from build123d import *

# Parameters (mm, degrees)
EXTRUDE_1_DEPTH     = 38
SKETCH_2_R          = 5
SKETCH_2_W          = 10
SKETCH_2_H          = 19
CUT_EXTRUDE_1_DEPTH = 8
SKETCH_3_W          = 4
SKETCH_3_H          = 4
CUT_EXTRUDE_2_DEPTH = 51.970579749
CUT_EXTRUDE_3_DEPTH = 65.567793829


with BuildPart() as part:
    # Эскиз1 → Бобышка-Вытянуть1 (new body)
    with BuildSketch(Plane.XY):
        Polygon((-5, 0), (-25, 0), (-25, -15), (25, -15), (25, 15), (12, -8), (-5, -8), align=None)
    extrude(amount=EXTRUDE_1_DEPTH)

    # Эскиз2 → Вырез-Вытянуть1 (cut)
    with BuildSketch(Plane(origin=(0, 0, 0), x_dir=(1, 0, 0), z_dir=(0, 1, 0))):
        with Locations((-25, -9.5)):
            Circle(SKETCH_2_R)
        with Locations((-10, -28.5)):
            Rectangle(SKETCH_2_W, SKETCH_2_H)
    extrude(amount=-CUT_EXTRUDE_1_DEPTH, mode=Mode.SUBTRACT)

    # Эскиз3 → Вырез-Вытянуть2 (cut, through all)
    with BuildSketch(Plane(origin=(0, -8, 0), x_dir=(1, 0, 0), z_dir=(0, 1, 0))):
        with Locations((-25, -9.5)):
            Rectangle(SKETCH_3_W, SKETCH_3_H)
        Polygon((1.350852961, -27), (7.701705922, -38), (-5, -38), align=None)
    extrude(amount=-CUT_EXTRUDE_2_DEPTH, mode=Mode.SUBTRACT)

    # Эскиз4 → Вырез-Вытянуть3 (cut, through all)
    with BuildSketch(Plane(origin=(25, 0, 0), x_dir=(0, 0, -1), z_dir=(1, 0, 0))):
        Polygon((-8, 15), (-28, 15), (-28, 5), (-8, 5), (-8, 10), (0, 10), (0, 15), align=None)
    extrude(amount=-CUT_EXTRUDE_3_DEPTH, mode=Mode.SUBTRACT)


solid = part.part
Design review of the part built by this model. Coordinates are the model's own, in mm. A direction names the side the tool comes from. Coordinates: 2 decimals unless noted, no trailing zeros. Order: outer loops, then holes, each group sorted by start corner. A loop starts at its lowest first (then second) coordinate and runs counter-clockwise, first axis right, second up. Notation, with made-up numbers: M 46,4 L 82,4 A20 ccw 82,23 Z; hole C 1.5,54.25 d8. An arc over 180 degrees is marked long. Use a Markdown table: item, result.
(1) For faces 4 (the flat face through (23, 7, 8)), 5 (the flat face through (17.15, 1.11, 18.73)), 6 (the flat face through (-10, -4, 19)), 7 (the flat face through (-24, -11, 11.5)), 8 (the cylindrical face through (-20, -3.9, 9.6)), list the 3-axis set-ups (+Z, -Z, +X, -X, +Y, -Y) from which the entire face can be reached by the end or side of a thin tool; tool diameter is ignored.
Worked answers:
| item | result |
|---|---|
| face 4 | +X, -X, +Y |
| face 5 | +Z, -Z, +Y |
| face 6 | +Z, +Y |
| face 7 | -X, +Y, -Y |
| face 8 | -X, +Y |
(2) For P1, Ø5.5, axis at x = -23, z = 7, coming from the +Y side; P2, Ø4.5, axis at x = 21.5, z = 14, coming from the +Y side; P3, Ø8, axis at x = 7, z = 11.5, coming from the +Y side, all flat-tipped, find the tip position at first contact; note any pin that passes through.
Worked answers:
| item | result |
|---|---|
| P1 | stops at y = 0 |
| P2 | stops at y = 5 |
| P3 | stops at y = -8 |
(3) Add section A-A (z = 33.5). Give the boundary of the cut face in (x, y).
Worked answers:
| item | result |
|---|---|
| outline | M -25,-15 L -2.4,-15 L -2.4,-8 L -15,-8 L -15,0 L -25,0 Z; M 5.1,-15 L 25,-15 L 25,15 L 12,-8 L 5.1,-8 Z |
(4) Wall thickness on probe 1 along Z at (x, y) = (-12, -4.5); probe 2 along Y at (x, z) = (5, 31); probe 3 along X at (y, z) = (-1.25, 28.5): over which ranges is each line inside the solid? List them lowest first.
Worked answers:
| item | result |
|---|---|
| probe 1 | z = 0 to 19 |
| probe 2 | y = -15 to -8 |
| probe 3 | x = -25 to -15, 15.82 to 25 |
(5) Add section C-C (z = 9.5). Give the boundary of the cut face in (x, y).
Worked answers:
| item | result |
|---|---|
| outline | M -23,-15 L 25,-15 L 25,5 L 19.35,5 L 12,-8 L -5,-8 L -5,0 L -20,0 L -20,-8 L -23,-8 Z |
(6) Add section B-B (y = -5.5). Give the boundary of the cut face in (x, z).
Worked answers:
| item | result |
|---|---|
| outline | M -25,0 L -5,0 L -5,19 L -15,19 L -15,38 L -25,38 L -25,14.5 A5 cw -25,4.5 Z; M 13.41,0 L 25,0 L 25,38 L 13.41,38 Z |
(7) Draft analysis for pull direction Z (two halves, no side actions). For faces 1 (the flat face through (-22.5, -8, 9.4)), 2 (the flat face through (-17, -9, 38)), 3 (the flat face through (-5, -4, 9)), state which applies: released by +Z, released by -Z, zero draft, split by the parting line, or undercut.
Worked answers:
| item | result |
|---|---|
| face 1 | undercut |
| face 2 | released by +Z |
| face 3 | zero draft |
(8) Add section D-D (y = -10.5). Give the boundary of the cut face in (x, z), then the cut area to 3 significant figures.
Worked answers:
| item | result |
|---|---|
| outline | M -25,0 L 25,0 L 25,38 L 7.7,38 L 1.35,27 L -5,38 L -25,38 L -25,11.5 L -23,11.5 L -23,7.5 L -25,7.5 Z |
| area | 1,820 mm2 |
